Design review of the part built by this model. Coordinates are the model's own, in mm. Face numbers are marked on the shaded views. A direction names the side the tool comes from. Coordinates: 2 decimals unless noted, no trailing zeros. Loops run counter-clockwise (first coordinate to the right, second up) from the corner with the lowest first, then second, coordinate; pieces in that order, holes last. Notation, with made-up numbers: M -1.75,28 L 33.25,28 A32 ccw 33.25,59 Z; hole C 16,20.25 d4. An arc over 180 degrees is marked long. Answer as a JSON object with one key per item and string values. Group by question number.
1. To check wall thickness, follow probe 1 along Y at (x, z) = (27, -16.5); probe 2 along X at (y, z) = (-1.5, -27.5); probe 3 along Y at (x, z) = (0, -19). State the ranges of each line that lie inside material, in increasing order.
2. Draft analysis for pull direction X (two halves, no side actions). For the marked faces 1, 2, 3 and 4, state which applies: +X half, -X half, draft (parallel to the pull), parting line (faces both ways), or undercut.
3. Machinability: for the marked faces 5, 6 and 7, which of the approach directions +Z, -Z, +X, -X, +Y, -Y give a long, thin tool a straight path to every point of the face, cutting with its end or side? Answer none if there is none.
4. Consider section D-D (y = 7). State the section outline as (x, z) points (3 decimals).
5. Consider section B-B (y = -12.5). State the section outline as (x, z) points.
6. Consider section C-C (z = -74). State the section outline as (x, y) points.
7. Insertion check: pin 1 (10 mm diameter, centred on x = 16.5, y = -3.5, fed in from +Z); pin 2 (3 mm diameter, centred on x = 56, y = 6, fed in from -Z); pin 3 (2.5 mm diameter, centred on x = 38, z = -21, fed in from +Y); pin 4 (6.5 mm diameter, centred on y = -5.5, z = -18.5, fed in from +X). Each pin has a flat end and moves straight along its axis. Give the tip position at first contact, or say it passes through.
8. Consider section A-A (x = 43.5). State the section outline as (y, z) points.
from build123d import *

# Parameters (mm, degrees)
SKETCH1_R               = 5.35
BOSS_EXTRUDE2_DEPTH     = 7
BOSS_EXTRUDE3_START     = 8
SKETCH3_R               = 5.35
BOSS_EXTRUDE3_DEPTH     = 8
BOSS_EXTRUDE4_DEPTH     = 3
FILLET1_R               = 1
CHAMFER1_SIZE           = 10
CHAMFER2_SIZE           = 5
CUT_EXTRUDE1_DEPTH      = 67.560662475
CUT_EXTRUDE1_DEPTH_BACK = 67.560662475
SKETCH5_W               = 31.474956737
SKETCH5_H               = 3.5
SKETCH5_H_2             = 8
CHAMFER3_SIZE           = 7
SKETCH6_R               = 11
BOSS_EXTRUDE5_DEPTH     = 5
SKETCH8_W               = 3
SKETCH8_H               = 7.519820499
SKETCH8_H_2             = 11.230179501
BOSS_EXTRUDE6_DEPTH     = 5
SKETCH9_R               = 3.5
BOSS_EXTRUDE7_DEPTH     = 68
CUT_EXTRUDE2_REACH      = 124.259
SKETCH10_W              = 8
SKETCH10_H              = 4


# Some blends are built 0.0001 mm under size
with BuildPart() as part:
    # Sketch1 → Boss-Extrude2 (new body)
    with BuildSketch(Plane.XY):
        Polygon((-19.503784034, -20), (19.503784034, -20), (19.503784034, -18.25), (62.978740771, -18.25), (62.978740771, 13), (19.503784034, 13), (19.503784034, 20), (-19.503784034, 20), align=None)
        Circle(SKETCH1_R, mode=Mode.SUBTRACT)
    extrude(amount=-BOSS_EXTRUDE2_DEPTH)

    # Sketch3 → Boss-Extrude3 (add)
    with BuildSketch(Plane.XY.offset(BOSS_EXTRUDE3_START)):
        with BuildLine():
            Line((7.668115805, 5.35), (62.978740771, 5.35))
            Line((62.978740771, 5.35), (62.978740771, 9.35))
            Line((62.978740771, 9.35), (0, 9.35))
            ThreePointArc((0, 9.35), (-9.35, 0), (0, -9.35))
            Line((0, -9.35), (62.978740771, -9.35))
            Line((62.978740771, -9.35), (62.978740771, -5.35))
            Line((62.978740771, -5.35), (7.668115805, -5.35))
            ThreePointArc((7.668115805, -5.35), (9.35, 0), (7.668115805, 5.35))
        make_face()
        Circle(SKETCH3_R, mode=Mode.SUBTRACT)
    extrude(amount=-BOSS_EXTRUDE3_DEPTH)

    # Sketch4 → Boss-Extrude4 (add)
    with BuildSketch(Plane.XY):
        with BuildLine():
            Line((0, -18.25), (62.978740771, -18.25))
            Line((62.978740771, -18.25), (62.978740771, -16.25))
            Line((62.978740771, -16.25), (8.306623863, -16.25))
            Line((8.306623863, -16.25), (0, -16.25))
            ThreePointArc((0, -16.25), (-16.25, 0), (0, 16.25))
            Line((0, 16.25), (0, 18.25))
            ThreePointArc((0, 18.25), (-18.25, 0), (0, -18.25))
        make_face()
    extrude(amount=BOSS_EXTRUDE4_DEPTH)

    # Fillet1
    fillet1_edges = [part.edges().sort_by_distance(p)[0] for p in [
        (0, 16.25, 1.5),
        (0, 18.25, 1.5),
    ]]
    fillet(fillet1_edges, radius=FILLET1_R - 0.0001)  # a hair under: the kernel refuses the full size

    # Chamfer1
    # the kernel refuses this chamfer: 10 mm, written as the material it takes off along each edge
    with BuildSketch(Plane(origin=(19.503784034, -20, 25.71682988), x_dir=(0.027495876610586317, 0.9996219169112968, 0), z_dir=(0, 0, -1))) as chamfer1_piece_1_section:
        Polygon((CHAMFER1_SIZE * 0.999621916911, -CHAMFER1_SIZE * 0.0274958766106), (-CHAMFER1_SIZE * 0.0274958766106, -CHAMFER1_SIZE * 0.999621916911), (0, 0), align=None)
    chamfer1_piece_1 = extrude(amount=58.433659759, mode=Mode.PRIVATE)
    chamfer1_piece_1 = split(chamfer1_piece_1, bisect_by=Plane(origin=(14.814200223, -18.25, -3.5), z_dir=(0, -1, 0)), keep=Keep.TOP, mode=Mode.PRIVATE)
    add(chamfer1_piece_1, mode=Mode.SUBTRACT)

    # Chamfer2
    chamfer2_edges = [part.edges().sort_by_distance(p)[0] for p in [
        (-19.503784034, -20, -3.5),
        (-19.503784034, 20, -3.5),
    ]]
    chamfer(chamfer2_edges, length=CHAMFER2_SIZE)

    # Sketch5 → Cut-Extrude1 (cut, two sides: drawn at the far end of the back side and taken through both)
    with BuildSketch(Plane.XY.offset(-CUT_EXTRUDE1_DEPTH_BACK)):
        with Locations((40.241262403, 3.6)):
            Rectangle(SKETCH5_W, SKETCH5_H)
        with Locations((40.241262403, -7.15)):
            Rectangle(SKETCH5_W, SKETCH5_H_2)
    extrude(amount=CUT_EXTRUDE1_DEPTH + CUT_EXTRUDE1_DEPTH_BACK, mode=Mode.SUBTRACT)

    # Chamfer3
    chamfer3_edges = [part.edges().sort_by_distance(p)[0] for p in [
        (19.503784034, 20, -3.5),
    ]]
    chamfer(chamfer3_edges, length=CHAMFER3_SIZE - 0.0001)  # a hair under: the kernel refuses the full size


with BuildPart() as body_2:
    # Mirror9: mirrored copy
    add(part.part.mirror(Plane.XY.offset(-10)))

    # Sketch6 → Boss-Extrude5 (add)
    with BuildSketch(Plane.XY.offset(-13)):
        Circle(SKETCH6_R)
    extrude(amount=BOSS_EXTRUDE5_DEPTH)

    # Sketch8 → Boss-Extrude6 (add)
    with BuildSketch(Plane(origin=(62.978740771, 0, 0), x_dir=(0, 0, -1), z_dir=(1, 0, 0))):
        with Locations((16.5, 6.240089751)):
            Rectangle(SKETCH8_W, SKETCH8_H)
        with Locations((16.5, -9.13491025)):
            Rectangle(SKETCH8_W, SKETCH8_H_2)
    extrude(amount=BOSS_EXTRUDE6_DEPTH)

    # Sketch9 → Boss-Extrude7 (add)
    with BuildSketch(Plane(origin=(0, 0, -20), x_dir=(-1, 0, 0), z_dir=(0, 0, -1))):
        with Locations((-20.003784034, 0)):
            Circle(SKETCH9_R)
    extrude(amount=BOSS_EXTRUDE7_DEPTH)

    # Sketch10 → Cut-Extrude2 (cut, up to next)
    with BuildSketch(Plane(origin=(62.978740771, 0, 0), x_dir=(0, 0, -1), z_dir=(1, 0, 0)), mode=Mode.PRIVATE) as cut_extrude2_sk1:
        with Locations((24, -7.35)):
            Rectangle(SKETCH10_W, SKETCH10_H)
    cut_extrude2_tool1 = extrude(cut_extrude2_sk1.sketch, amount=-CUT_EXTRUDE2_REACH, mode=Mode.PRIVATE) & body_2.part
    add(cut_extrude2_tool1.solids().sort_by_distance((62.978741, -7.35, -24))[0], mode=Mode.SUBTRACT)


solid = body_2.part
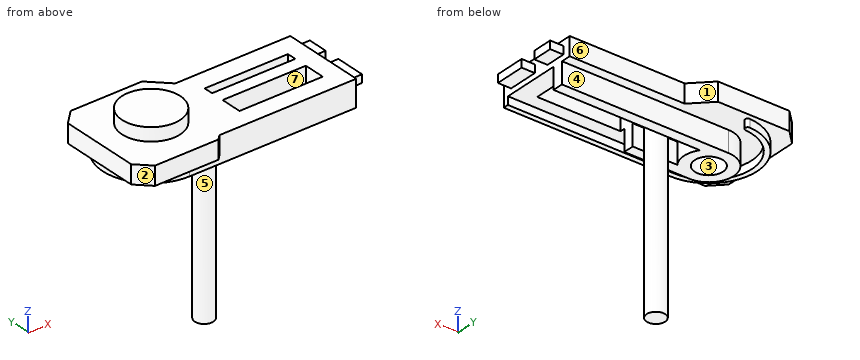
Findings below:
{
 "1": {"probe 1": "y = -18.25 to -11.15, -3.15 to 1.85, 5.35 to 13", "probe 2": "x = -9.23 to -5.14, 5.14 to 9.23, 16.84 to 23.17", "probe 3": "y = -20 to -5.35, 5.35 to 20"},
 "2": {"face 1": "+X half", "face 2": "-X half", "face 3": "undercut", "face 4": "draft"},
 "3": {"face 5": "-Z", "face 6": "+Z, -Z, +X, +Y", "face 7": "+Z, -Z"},
 "4": {"outline": "M -19.504,-20 L -16.854,-20 L -16.854,-23 L -14.665,-23 L -14.665,-20 L -6.199,-20 L -6.199,-28 L 62.979,-28 L 62.979,-18 L 67.979,-18 L 67.979,-15 L 62.979,-15 L 62.979,-13 L 8.485,-13 L 8.485,-8 L -8.485,-8 L -8.485,-13 L -19.504,-13 Z"},
 "5": {"outline": "M -19.5,-20 L -13.3,-20 L -13.3,-23 L -10.38,-23 L -10.38,-20 L 62.98,-20 L 62.98,-18 L 67.98,-18 L 67.98,-15 L 62.98,-15 L 62.98,-13 L -19.5,-13 Z"},
 "6": {"outline": "C 20,0 d7"},
 "7": {"pin 1": "stops at z = -13", "pin 2": "stops at z = -28", "pin 3": "stops at y = 13", "pin 4": "stops at x = 67.98"},
 "8": {"outline": "M -18.25,-23 L -16.25,-23 L -16.25,-20 L -11.15,-20 L -11.15,-13 L -18.25,-13 Z; M -3.15,-20 L 1.85,-20 L 1.85,-13 L -3.15,-13 Z; M 5.35,-28 L 9.35,-28 L 9.35,-20 L 13,-20 L 13,-13 L 5.35,-13 Z"}
}
